Design review of the part shown in the three views and the two pictorial views. Dimensions are in mm from the part's minimum x, y and z. A direction names the side the tool comes from. Round coordinates to 2 decimals unless told otherwise and drop trailing zeros. Write each loop counter-clockwise with the first axis right and the second up, starting at its lowest first coordinate (ties: lowest second). Pieces come first, ordered by that corner, then holes. Notation, with made-up numbers: (61, -36) -> (77, -36) arc R20 cw to (77, -21) -> close; hole circle Ø2 at (19, 59.25). An arc over 180 degrees is marked (long way). Answer as a JSON object with one key per item and string values. Group by question number.
1) Mouldability with a two-part tool opening along X and no side actions: class the marked faces 3, 4 and 5 as pulls with the +X half, pulls with the -X half, needs draft (parallel to the pull), parting line crosses it, or undercut.
2) We need section C-C, the plane z = 13.75. Write out the cut boundary in (x, y).
3) Insertion check: pin 1 Ø2.5 at (x, y) = (45, 47) entering from -Z; pin 2 Ø4 at (y, z) = (30.5, 7.5) entering from -X; pin 3 Ø4 at (x, y) = (17, 48.5) entering from +Z. Each pin has a flat end and moves straight along its axis. Give the tip position at first contact, or say it passes through.
4) To check wall thickness, follow probe 1 along X at (y, z) = (26, 10); probe 2 along X at (y, z) = (47, 5.25); probe 3 along Y at (x, z) = (36.5, 5.25). State the ranges of each line that lie inside material, in increasing order. Write a range as [from, to].
5) Machinability: for the marked faces 1 and 2, which of the approach directions +Z, -Z, +X, -X, +Y, -Y give a long, thin tool a straight path to every point of the face, cutting with its end or side? Answer none if there is none.
6) We need section A-A, the plane y = 35.5. Write out the cut boundary in (x, z), then the cut area to 3 significant figures.
7) We need section D-D, the plane x = 18. Write out the cut boundary in (y, z), then the cut area to 3 significant figures.
8) We need section B-B, the plane x = 30. Write out the cut boundary in (y, z), then the cut area to 3 significant figures.
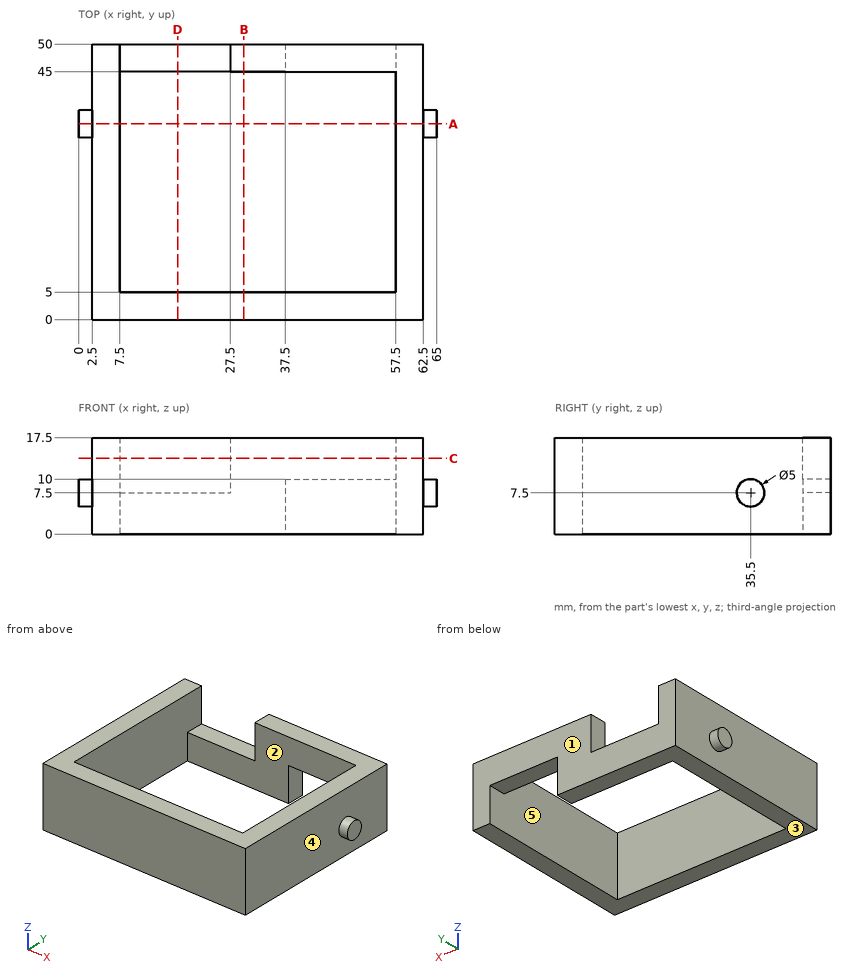
Here are the results:
{
 "1": {"face 3": "needs draft", "face 4": "pulls with the +X half", "face 5": "undercut"},
 "2": {"outline": "(2.5, 0) -> (62.5, 0) -> (62.5, 50) -> (27.5, 50) -> (27.5, 45) -> (57.5, 45) -> (57.5, 5) -> (7.5, 5) -> (7.5, 50) -> (2.5, 50) -> close"},
 "3": {"pin 1": "stops at z = 10", "pin 2": "stops at x = 2.5", "pin 3": "stops at z = 7.5"},
 "4": {"probe 1": "x = [2.5, 7.5], [57.5, 62.5]", "probe 2": "x = [2.5, 37.5], [57.5, 62.5]", "probe 3": "y = [0, 5], [45, 50]"},
 "5": {"face 1": "+Z, -Z, +X, -X, +Y", "face 2": "+Z, -Z"},
 "6": {"outline": "(0, 5) -> (2.5, 5) -> (2.5, 0) -> (7.5, 0) -> (7.5, 17.5) -> (2.5, 17.5) -> (2.5, 10) -> (0, 10) -> close; (57.5, 0) -> (62.5, 0) -> (62.5, 5) -> (65, 5) -> (65, 10) -> (62.5, 10) -> (62.5, 17.5) -> (57.5, 17.5) -> close", "area": "200 mm^2"},
 "7": {"outline": "(0, 0) -> (5, 0) -> (5, 17.5) -> (0, 17.5) -> close; (45, 0) -> (50, 0) -> (50, 7.5) -> (45, 7.5) -> close", "area": "125 mm^2"},
 "8": {"outline": "(0, 0) -> (5, 0) -> (5, 17.5) -> (0, 17.5) -> close; (45, 0) -> (50, 0) -> (50, 17.5) -> (45, 17.5) -> close", "area": "175 mm^2"}
}
